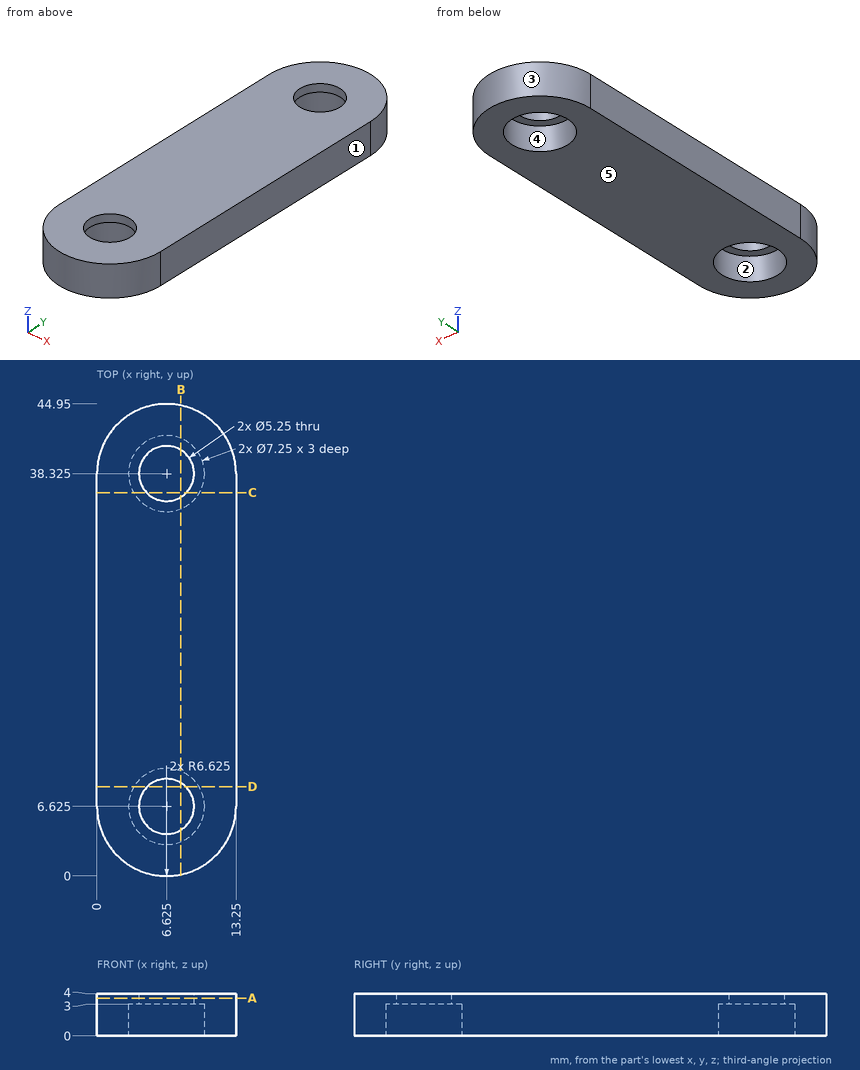
Job drawing, mm, ordinate dimensions from the low corner. One solid piece. A direction names the side the tool comes from. Coordinates: 2 decimals unless noted, no trailing zeros. Write each loop counter-clockwise with the first axis right and the second up, starting at its lowest first coordinate (ties: lowest second). Pieces come first, ordered by that corner, then holes. Notation, with made-up numbers: M 47.25,-2.5 L 88.25,-2.5 A20 cw 88.25,9.5 Z; hole C 40.5,20 d4. An arc over 180 degrees is marked long. Answer as a JSON object with one key per item and string values. Group by question number.
1) Saw through at C-C (y = 36.5). Write the cut outline in (x, z).
2) Mould opens along Y. For the marked faces 1, 2 and 3 say: +Y half, -Y half, draft (parallel to the pull), parting line (faces both ways), or undercut.
3) Saw through at D-D (y = 8.5). Write the cut outline in (x, z), plus the area to 3 significant figures.
4) Saw through at B-B (x = 8). Write the cut outline in (y, z).
5) Wall check: line 1 (Y direction, x = 6.75, z = 0.6); line 2 (Y direction, x = 9.25, z = 0.5) (3 decimals); line 3 (X direction, y = 37.5, z = 3.05). Give the ranges that are in metal, low to high. Write a range as from..to.
6) Tool access for the marked faces 4 and 5: list every direction of +Z, -Z, +X, -X, +Y, -Y with a clear straight run to the whole face (end or side of a thin tool).
7) Saw through at A-A (z = 3.6). Write the cut outline in (x, y) (3 decimals), plus the area to 3 significant figures.
8) Pin check, flat tips, straight feed: pin 1 Ø2 at (x, y) = (7.5, 6) entering from -Z; pin 2 Ø2 at (x, z) = (8, 2.5) entering from -Y; pin 3 Ø2 at (x, z) = (8.5, 3) entering from +Y. Stop position of each tip, or through.
Values follow:
{
 "1": {"outline": "M 0,0 L 3.49,0 L 3.49,3 L 4.74,3 L 4.74,4 L 0,4 Z; M 8.51,3 L 9.76,3 L 9.76,0 L 13.25,0 L 13.25,4 L 8.51,4 Z"},
 "2": {"face 1": "draft", "face 2": "undercut", "face 3": "+Y half"},
 "3": {"outline": "M 0,0 L 3.52,0 L 3.52,3 L 4.79,3 L 4.79,4 L 0,4 Z; M 8.46,3 L 9.73,3 L 9.73,0 L 13.25,0 L 13.25,4 L 8.46,4 Z", "area": "30.7 mm2"},
 "4": {"outline": "M 0.14,0 L 3.27,0 L 3.27,3 L 4.39,3 L 4.39,4 L 0.14,4 Z; M 8.86,3 L 9.98,3 L 9.98,0 L 34.97,0 L 34.97,3 L 36.09,3 L 36.09,4 L 8.86,4 Z; M 40.56,3 L 41.68,3 L 41.68,0 L 44.81,0 L 44.81,4 L 40.56,4 Z"},
 "5": {"line 1": "y = 0..3, 10.25..34.7, 41.95..44.95", "line 2": "y = 0.542..4.125, 9.125..35.825, 40.825..44.408", "line 3": "x = 0..4.13, 9.12..13.25"},
 "6": {"face 4": "-Z", "face 5": "-Z, +X, -X, +Y, -Y"},
 "7": {"outline": "M 0,6.625 A6.625 ccw 13.25,6.625 L 13.25,38.325 A6.625 ccw 0,38.325 Z; hole C 6.625,6.625 d5.25; hole C 6.625,38.325 d5.25", "area": "515 mm2"},
 "8": {"pin 1": "passes through", "pin 2": "stops at y = 0.01", "pin 3": "stops at y = 44.89"}
}
